```python
from build123d import *

# Parameters (mm, degrees)
F1_DEPTH = 6


with BuildPart() as f1:
    # F0 (on Top) → F1 (new body)
    with BuildSketch(Plane.XY):
        with BuildLine():
            ThreePointArc((243.905, 260.5), (249, 265.595), (254.095, 260.5))
            Line((254.095, 260.5), (254.095, -210.5))
            ThreePointArc((254.095, -210.5), (252.602709, -214.102709), (249, -215.595))
            Line((249, -215.595), (0, -215.595))
            Line((0, -215.595), (-249, -215.595))
            ThreePointArc((-249, -215.595), (-252.602709, -214.102709), (-254.095, -210.5))
            Line((-254.095, -210.5), (-254.095, 5))
            ThreePointArc((-254.095, 5), (-252.602709, 8.602709), (-249, 10.095))
            Line((-249, 10.095), (0, 10.095))
            Line((0, 10.095), (0, 10.116))
            Line((0, 10.116), (0, 10.725))
            Line((0, 10.725), (-249, 10.725))
            ThreePointArc((-249, 10.725), (-253.048186, 9.048186), (-254.725, 5))
            Line((-254.725, 5), (-254.725, -210.5))
            ThreePointArc((-254.725, -210.5), (-253.048186, -214.548186), (-249, -216.225))
            Line((-249, -216.225), (0, -216.225))
            Line((0, -216.225), (249, -216.225))
            ThreePointArc((249, -216.225), (253.048186, -214.548186), (254.725, -210.5))
            Line((254.725, -210.5), (254.725, 260.5))
            ThreePointArc((254.725, 260.5), (249, 266.225), (243.275, 260.5))
            Line((243.275, 260.5), (243.275, -5))
            ThreePointArc((243.275, -5), (242.037526, -7.987526), (239.050001, -9.224999))
            Line((239.050001, -9.224999), (236.658265, -9.224999))
            Line((236.658265, -9.224999), (0, -9.224999))
            Line((0, -9.224999), (0, -9.854999))
            Line((0, -9.854999), (239.050001, -9.854999))
            ThreePointArc((239.050001, -9.854999), (242.483004, -8.433003), (243.905, -5))
            Line((243.905, -5), (243.905, 260.5))
        make_face()
    extrude(amount=F1_DEPTH)


solid = f1.part
```
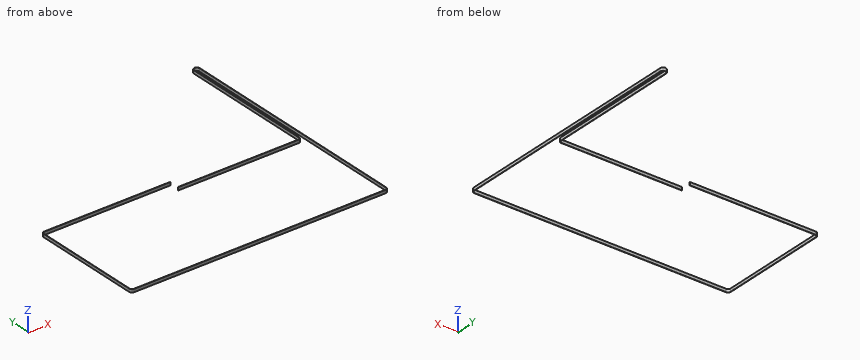
Can you work these out from the model? Positions are in its coordinate system, mm. Round coordinates to 2 decimals unless told otherwise and drop trailing zeros. Loops run counter-clockwise (first coordinate to the right, second up) from the corner with the lowest first, then second, coordinate; pieces in that order, holes last. Notation, with made-up numbers: (55.5, 27) -> (93.5, 27) arc R36 ccw to (93.5, 64) -> close; hole circle Ø6 at (-39, -16.75). An arc over 180 degrees is marked (long way). One line per item, written item: value. Start each with the question number.
1. If we section it at A-A, the plane x = -150: Write out the boundary of the cut face in (y, z) (3 decimals).
2. If I drill on probe 1 along X at (y, z) = (6, 0.45) (3 decimals); probe 2 along Y at (x, z) = (-109, 4.85) (3 decimals); probe 3 along Y at (x, z) = (43.5, 1.4) (3 decimals), over which ranges is the centre line in solid material (lowest first)?
3. If we section it at B-B, the plane y = 50: Write out the boundary of the cut face in (x, z) (3 decimals).
4. For pin 1 (1.8 mm diameter, centred on y = 99.5, z = 2, fed in from -X) (3 decimals); pin 2 (3 mm diameter, centred on x = -82.5, z = 4, fed in from +Y) (3 decimals); pin 3 (1.8 mm diameter, centred on x = 140, z = 2, fed in from +Y) (3 decimals), each with a flat end and sliding along its axis, tell me the tip position at first contact or that it passes through.
5. If we section it at C-C, the plane z = 3.6: Write out the boundary of the cut face in (x, y) (3 decimals), then the cut area to 3 significant figures.
Calculated:
1. outline: (-216.225, 0) -> (-215.595, 0) -> (-215.595, 6) -> (-216.225, 6) -> close; (10.095, 0) -> (10.725, 0) -> (10.725, 6) -> (10.095, 6) -> close
2. probe 1: x = -254.637 to -253.996, 243.275 to 243.905, 254.095 to 254.725
2. probe 2: y = -216.225 to -215.595, 10.095 to 10.725
2. probe 3: y = -216.225 to -215.595, -9.855 to -9.225
3. outline: (243.275, 0) -> (243.905, 0) -> (243.905, 6) -> (243.275, 6) -> close; (254.095, 0) -> (254.725, 0) -> (254.725, 6) -> (254.095, 6) -> close
4. pin 1: stops at x = 243.275
4. pin 2: stops at y = 10.725
4. pin 3: stops at y = -9.225
5. outline: (-254.725, -210.5) arc R5.725 ccw to (-249, -216.225) -> (249, -216.225) arc R5.725 ccw to (254.725, -210.5) -> (254.725, 260.5) arc R5.725 ccw to (243.275, 260.5) -> (243.275, -5) arc R4.225 cw to (239.05, -9.225) -> (0, -9.225) -> (0, -9.855) -> (239.05, -9.855) arc R4.855 ccw to (243.905, -5) -> (243.905, 260.5) arc R5.095 cw to (254.095, 260.5) -> (254.095, -210.5) arc R5.095 cw to (249, -215.595) -> (-249, -215.595) arc R5.095 cw to (-254.095, -210.5) -> (-254.095, 5) arc R5.095 cw to (-249, 10.095) -> (0, 10.095) -> (0, 10.725) -> (-249, 10.725) arc R5.725 ccw to (-254.725, 5) -> close
5. area: 1,250 mm²
